Build history of the part. All positions in model axes, mm. A direction names the side the tool comes from. Round coordinates to 2 decimals unless told otherwise and drop trailing zeros. Loops run counter-clockwise (first coordinate to the right, second up) from the corner with the lowest first, then second, coordinate; pieces in that order, holes last. Notation, with made-up numbers: M 52.5,31.25 L 57.5,31.25 A17 ccw 57.5,63.25 Z; hole C 23.5,27.25 d11. An arc over 180 degrees is marked long. Use one line per item in the form item = value. Start each with the question number.
```python
from build123d import *

# Parameters (mm, degrees)
BOSS_EXTRUDE1_DEPTH     = 38.1
CUT_EXTRUDE1_REACH      = 79.512
SKETCH2_R               = 3.175
CUT_EXTRUDE2_REACH      = 79.512
SKETCH4_R               = 3.175
CHAMFER1_SIZE           = 2.54
CUT_EXTRUDE3_DEPTH      = 78.51162816
CUT_EXTRUDE3_DEPTH_BACK = 78.51162816


with BuildPart() as part:
    # Sketch1 → Boss-Extrude1 (new body)
    with BuildSketch(Plane(origin=(0, 0, 0), x_dir=(1, 0, 0), z_dir=(0, 1, 0))):
        Polygon((0, 0), (0, 50.8), (44.45, 50.8), (44.45, 46.0375), (4.7625, 46.0375), (4.7625, 0), align=None)
    extrude(amount=BOSS_EXTRUDE1_DEPTH)

    # Sketch2 → Cut-Extrude1 (cut, up to next)
    with BuildSketch(Plane(origin=(0, 0, -50.8), x_dir=(-1, 0, 0), z_dir=(0, 0, -1)), mode=Mode.PRIVATE) as cut_extrude1_sk1:
        with Locations((-12.7, 21.20738686)):
            Circle(SKETCH2_R)
    cut_extrude1_tool1 = extrude(cut_extrude1_sk1.sketch, amount=-CUT_EXTRUDE1_REACH, mode=Mode.PRIVATE) & part.part
    # Sketch2 → Cut-Extrude1 (cut, up to next)
    with BuildSketch(Plane(origin=(0, 0, -50.8), x_dir=(-1, 0, 0), z_dir=(0, 0, -1)), mode=Mode.PRIVATE) as cut_extrude1_sk2:
        with Locations((-31.75, 16.102954744)):
            Circle(SKETCH2_R)
    cut_extrude1_tool2 = extrude(cut_extrude1_sk2.sketch, amount=-CUT_EXTRUDE1_REACH, mode=Mode.PRIVATE) & part.part
    add(cut_extrude1_tool1.solids().sort_by_distance((12.7, 21.207387, -50.8))[0], mode=Mode.SUBTRACT)
    add(cut_extrude1_tool2.solids().sort_by_distance((31.75, 16.102955, -50.8))[0], mode=Mode.SUBTRACT)

    # Sketch4 → Cut-Extrude2 (cut, up to next)
    with BuildSketch(Plane.ZY, mode=Mode.PRIVATE) as cut_extrude2_sk1:
        with Locations((-12.7, 19.05)):
            Circle(SKETCH4_R)
    cut_extrude2_tool1 = extrude(cut_extrude2_sk1.sketch, amount=-CUT_EXTRUDE2_REACH, mode=Mode.PRIVATE) & part.part
    # Sketch4 → Cut-Extrude2 (cut, up to next)
    with BuildSketch(Plane.ZY, mode=Mode.PRIVATE) as cut_extrude2_sk2:
        with Locations((-38.1, 19.05)):
            Circle(SKETCH4_R)
    cut_extrude2_tool2 = extrude(cut_extrude2_sk2.sketch, amount=-CUT_EXTRUDE2_REACH, mode=Mode.PRIVATE) & part.part
    add(cut_extrude2_tool1.solids().sort_by_distance((0, 19.05, -12.7))[0], mode=Mode.SUBTRACT)
    add(cut_extrude2_tool2.solids().sort_by_distance((0, 19.05, -38.1))[0], mode=Mode.SUBTRACT)

    # Chamfer1
    chamfer1_edges = [part.edges().sort_by_distance(p)[0] for p in [
        (0, 19.05, -15.875),
        (0, 19.05, -41.275),
    ]]
    chamfer(chamfer1_edges, length=CHAMFER1_SIZE)

    # Sketch5 → Cut-Extrude3 (cut, two sides: drawn at the far end of the back side and taken through both)
    with BuildSketch(Plane(origin=(0, 0, -50.8), x_dir=(-1, 0, 0), z_dir=(0, 0, -1)).offset(-CUT_EXTRUDE3_DEPTH_BACK)):
        Polygon((28.817809215, -90.851713823), (-31.75, 0), (-44.45, 19.05), (-105.017809215, 109.901713823), (-286.721236861, -11.233904608), (-152.88561843, -211.987332253), align=None)
    extrude(amount=CUT_EXTRUDE3_DEPTH + CUT_EXTRUDE3_DEPTH_BACK, mode=Mode.SUBTRACT)


solid = part.part
```
Q1. Pull direction Z, two halves, no side cores. Call faces 3 (the face through (25, 19, -46.038)), 4 (the face through (22, 19, -50.8)), 5 (the face through (4, 38.1, -35)), 6 (the face through (2.417, 19.195, -15.995)): pulls with the +Z half, pulls with the -Z half, needs draft (parallel to the pull), parting line crosses it, or undercut.
Q2. Tool access for faces 1 (the face through (4.762, 19, -23)), 2 (the face through (2, 19, 0)): list every direction of +Z, -Z, +X, -X, +Y, -Y with a clear straight run to the whole face (end or side of a thin tool).
Q3. Saw through at C-C (y = 31). Give the cut face in (x, z), and give its area (3 significant figures).
Q4. Saw through at A-A (z = -12.7). Give the cut face in (x, y) (1 decimal), and give its area (3 significant figures).
Q5. Drop flat-ended pins along their axis: P1, Ø7.5, axis at y = 19.05, z = -38.1, coming from the +X side; P2, Ø5.5, axis at x = 31.75, y = 16.1, coming from the -Z side. Give the stop position or say it passes through.
Q6. Saw through at D-D (x = 32.5). Give the cut face in (y, z) (1 decimal).
Q7. Wall check: probe 1 along Y at (x, z) = (3.45, -12.7) (3 decimals); probe 2 along Z at (x, y) = (42, 16); probe 3 along X at (y, z) = (11.5, -41.5). Give the ranges that are in metal, low to high.
Q8. Saw through at B-B (x = 12.7). Give the cut face in (y, z), and give its area (3 significant figures).
Filled in:
q1.face_3 = pulls with the +Z half
q1.face_4 = pulls with the -Z half
q1.face_5 = needs draft
q1.face_6 = undercut
q2.face_1 = +Z, +X, +Y, -Y
q2.face_2 = +Z, +X, -X, +Y, -Y
q3.outline = M 0,-50.8 L 44.45,-50.8 L 44.45,-46.04 L 4.76,-46.04 L 4.76,0 L 0,0 Z
q3.area = 431 mm²
q4.outline = M 0,0 L 4.8,0 L 4.8,15.9 L 2.5,15.9 L 0,13.3 Z; M 0,24.8 L 2.5,22.2 L 4.8,22.2 L 4.8,38.1 L 0,38.1 Z
q4.area = 145 mm²
q5.P1 = 4.76
q5.P2 = through
q6.outline = M 1.1,-50.8 L 13,-50.8 L 13,-46 L 1.1,-46 Z; M 19.2,-50.8 L 38.1,-50.8 L 38.1,-46 L 19.2,-46 Z
q7.probe_1 = 0 to 15.875, 22.225 to 38.1
q7.probe_2 = -50.8 to -46.04
q7.probe_3 = 0 to 4.76
q8.outline = M 0,-50.8 L 18.03,-50.8 L 18.03,-46.04 L 0,-46.04 Z; M 24.38,-50.8 L 38.1,-50.8 L 38.1,-46.04 L 24.38,-46.04 Z
q8.area = 151 mm²
